The figure shows three views and two pictorial views of one solid part (mm, origin at its lowest corner). Answer the questions. A direction names the side the tool comes from. Give positions to 0.01 mm unless a question says otherwise; leave off trailing zeros. Order: outer loops, then holes, each group sorted by start corner. A loop starts at its lowest first (then second) coordinate and runs counter-clockwise, first axis right, second up. Notation, with made-up numbers: M 15.5,33 L 37.5,33 A15 ccw 37.5,40 Z; hole C 73,2.25 d7. An arc over 180 degrees is marked long. One line per item, written item: value.
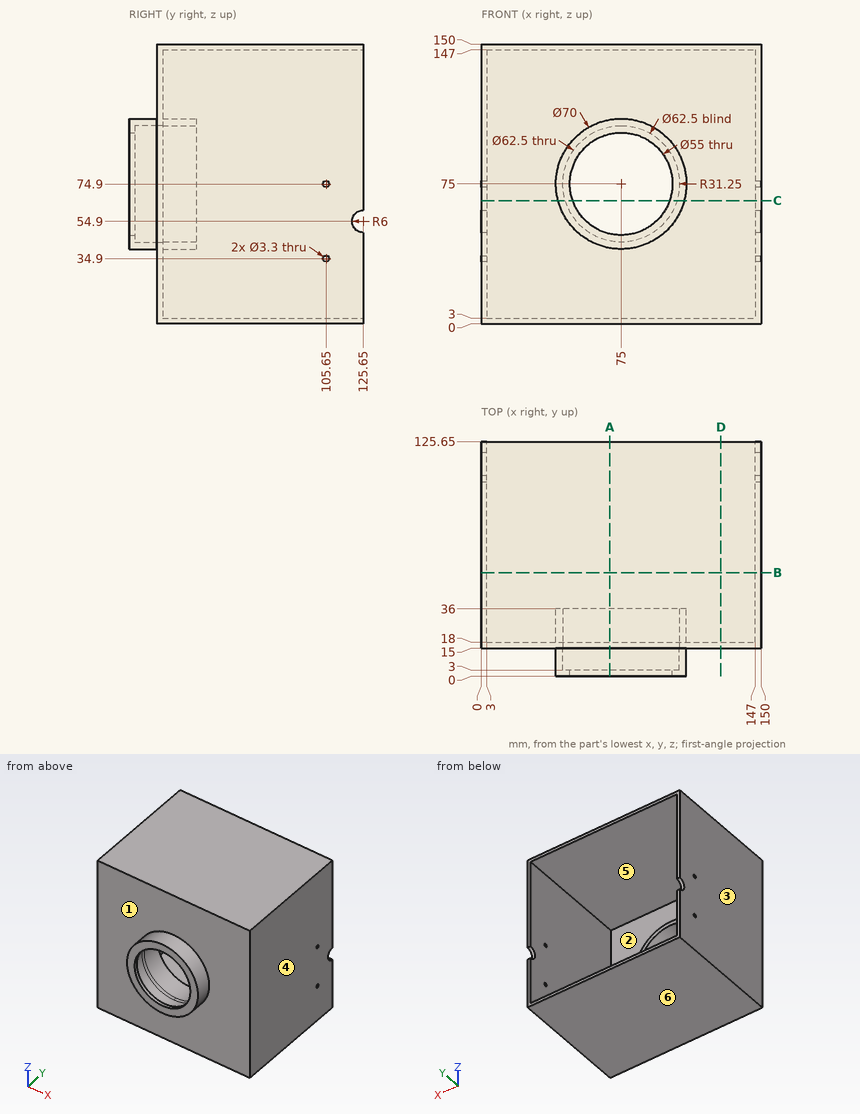
1) Which of the six approach directions +Z, -Z, +X, -X, +Y, -Y give full straight-line access (tool end or side, diameter ignored) to the marked faces 1, 2 and 3?
Reported:
face 1: -Y
face 2: +Y
face 3: +Z, -Z, -X, +Y, -Y
2) Consider probe 1 along Z at (x, y) = (148.25, 105.65); probe 2 along Z at (x, y) = (47.5, 61). Determine where each line is inside the solid, lowest interval first.
Reported:
probe 1: z = 0 to 33.25, 36.55 to 73.25, 76.55 to 150
probe 2: z = 0 to 3, 147 to 150
3) Determine the mould class of the marked faces 4, 5 and 6 for opening direction X: +X half, -X half, draft (parallel to the pull), parting line (faces both ways), or undercut.
Reported:
face 4: +X half
face 5: undercut
face 6: draft
4) Find section B-B, the plane y = 55.5. Write down the section's boundary in (x, z), plus the area to 3 significant figures.
Reported:
outline: M 0,0 L 150,0 L 150,150 L 0,150 Z; hole M 3,3 L 147,3 L 147,147 L 3,147 Z
area: 1,760 mm^2
5) Find section D-D, the plane x = 128.5. Write down the section's boundary in (y, z), plus the area to 3 significant figures.
Reported:
outline: M 15,0 L 125.65,0 L 125.65,3 L 18,3 L 18,147 L 125.65,147 L 125.65,150 L 15,150 Z
area: 1,100 mm^2
6) Each of these flat-tipped pins is pushed along its axis until it touches: pin 1 Ø4 at (y, z) = (111.5, 59.5) entering from -X; pin 2 Ø2.5 at (y, z) = (105.65, 74.9) entering from +X; pin 3 Ø5 at (x, z) = (114.5, 91.5) entering from -Y; pin 4 Ø21 at (x, z) = (89, 87.5) entering from +Y. Where does it stop, or does it pass through?
Reported:
pin 1: stops at x = 0
pin 2: passes through
pin 3: stops at y = 15
pin 4: stops at y = 3
7) Find section C-C, the plane z = 66. Write down the section's boundary in (x, y), plus the area to 3 significant figures.
Reported:
outline: M 0,15 L 41.18,15 L 41.18,0 L 49.01,0 L 49.01,3 L 45.07,3 L 45.07,36 L 41.18,36 L 41.18,18 L 3,18 L 3,125.65 L 0,125.65 Z; M 100.99,0 L 108.82,0 L 108.82,15 L 150,15 L 150,125.65 L 147,125.65 L 147,18 L 108.82,18 L 108.82,36 L 104.93,36 L 104.93,3 L 100.99,3 Z
area: 1,200 mm^2
8) Find section A-A, the plane x = 69. Write down the section's boundary in (y, z), plus the area to 3 significant figures.
Reported:
outline: M 0,40.52 L 15,40.52 L 15,0 L 125.65,0 L 125.65,3 L 18,3 L 18,40.52 L 36,40.52 L 36,44.33 L 3,44.33 L 3,48.16 L 0,48.16 Z; M 0,101.84 L 3,101.84 L 3,105.67 L 36,105.67 L 36,109.48 L 18,109.48 L 18,147 L 125.65,147 L 125.65,150 L 15,150 L 15,109.48 L 0,109.48 Z
area: 1,190 mm^2
